```python
from build123d import *

# Parameters (mm, degrees)
SKETCH_3_R               = 3
EXTRUDE_6_DEPTH          = 0.001
EXTRUDE_6_2_DEPTH        = 0.001
EXTRUDE_6_3_DEPTH        = 0.001
EXTRUDE_6_4_DEPTH        = 0.001
CUT_EXTRUDE_2_DEPTH      = 67.213034483
CUT_EXTRUDE_2_DEPTH_BACK = 67.213034483
SKETCH_11_R              = 2.25
EXTRUDE_7_DEPTH          = 2
EXTRUDE_7_DEPTH_BACK     = 0.801922547
SKETCH_14_R              = 10
CUT_EXTRUDE_3_DEPTH      = 3
SKETCH_12_4_R            = 10
EXTRUDE_10_DEPTH         = 44
SKETCH_20_W              = 40.801922547
SKETCH_20_H              = 50
CUT_EXTRUDE_6_DEPTH      = 60
SKETCH_21_W              = 44.801922547
SKETCH_21_H              = 50
EXTRUDE_11_DEPTH         = 2
SKETCH_23_W              = 4
SKETCH_23_H              = 35
EXTRUDE_12_DEPTH         = 35
CUT_EXTRUDE_7_DEPTH      = 75.778269065
SKETCH_25_R              = 0.75
CUT_EXTRUDE_8_DEPTH      = 84.687483396
FILLET_2_R               = 5
FILLET_3_R               = 5
FILLET_5_R               = 3
FILLET_6_R               = 3
FILLET_7_R               = 3
FILLET_8_R               = 3
SKETCH_26_R              = 2.75
CUT_EXTRUDE_9_DEPTH      = 100
SKETCH_27_R              = 10
SKETCH_27_R_2            = 7.5
EXTRUDE_13_DEPTH         = 5
SKETCH_28_R              = 10
SKETCH_28_R_2            = 7.5
EXTRUDE_14_DEPTH         = 5
CUT_EXTRUDE_10_DEPTH     = 86.331157337
CUT_EXTRUDE_11_DEPTH     = 86.331157337
CUT_EXTRUDE_12_DEPTH     = 86.331157337
EXTRUDE_15_DEPTH         = 50


with BuildPart() as part:
    # Sketch 3 → Extrude 6 (new body)
    with BuildSketch(Plane.XY):
        with Locations((60.266478541, 16.532501821)):
            Circle(SKETCH_3_R)
    extrude(amount=EXTRUDE_6_DEPTH)


with BuildPart() as body_2:
    # Sketch 3 → Extrude 6 2 (new body)
    with BuildSketch(Plane.XY):
        with Locations((60.266478541, 6.532501821)):
            Circle(SKETCH_3_R)
    extrude(amount=EXTRUDE_6_2_DEPTH)


with BuildPart() as body_3:
    # Sketch 3 → Extrude 6 3 (new body)
    with BuildSketch(Plane.XY):
        with Locations((10.766478541, 6.532501821)):
            Circle(SKETCH_3_R)
    extrude(amount=EXTRUDE_6_3_DEPTH)


with BuildPart() as body_4:
    # Sketch 3 → Extrude 6 4 (new body)
    with BuildSketch(Plane.XY):
        with Locations((10.766478541, 16.532501821)):
            Circle(SKETCH_3_R)
    extrude(amount=EXTRUDE_6_4_DEPTH)


with BuildPart() as cut_extrude_2_tool:
    # Sketch 11 → Cut-Extrude 2 (new, two sides: drawn at the far end of the back side and taken through both)
    with BuildSketch(Plane.XY.offset(0.001).offset(-CUT_EXTRUDE_2_DEPTH_BACK)):
        with Locations((10.766478541, 16.532501821)):
            Circle(SKETCH_11_R)
        with Locations((10.766478541, 6.532501821)):
            Circle(SKETCH_11_R)
        with Locations((60.266478541, 16.532501821)):
            Circle(SKETCH_11_R)
        with Locations((60.266478541, 6.532501821)):
            Circle(SKETCH_11_R)
    extrude(amount=CUT_EXTRUDE_2_DEPTH + CUT_EXTRUDE_2_DEPTH_BACK)


with BuildPart() as part_1:
    add(part.part)

    # Cut-Extrude 2: cut by cut_extrude_2_tool
    add(cut_extrude_2_tool.part, mode=Mode.SUBTRACT)



with BuildPart() as body_2_1:
    add(body_2.part)

    # Cut-Extrude 2: cut by cut_extrude_2_tool
    add(cut_extrude_2_tool.part, mode=Mode.SUBTRACT)


with BuildPart() as body_3_1:
    add(body_3.part)

    # Cut-Extrude 2: cut by cut_extrude_2_tool
    add(cut_extrude_2_tool.part, mode=Mode.SUBTRACT)


with BuildPart() as body_4_1:
    add(body_4.part)

    # Cut-Extrude 2: cut by cut_extrude_2_tool
    add(cut_extrude_2_tool.part, mode=Mode.SUBTRACT)


with BuildPart() as body_5:
    # Sketch 12 → Extrude 7 (new, two sides: drawn at the far end of the back side and taken through both)
    with BuildSketch(Plane.XY.offset(0.001).offset(-EXTRUDE_7_DEPTH_BACK)):
        Polygon((5.516478541, 26.532501821), (65.516478541, 26.532501821), (65.516478541, -23.467498179), (5.516478541, -23.467498179), (5.516478541, 1.532501821), align=None)
    extrude(amount=EXTRUDE_7_DEPTH + EXTRUDE_7_DEPTH_BACK)

    # Sketch 14 → Cut-Extrude 3 (cut)
    with BuildSketch(Plane(origin=(0, 0, -0.800922547), x_dir=(-1, 0, 0), z_dir=(0, 0, -1))):
        with Locations((-45.516478541, 11.532501821)):
            Circle(SKETCH_14_R)
    extrude(amount=-CUT_EXTRUDE_3_DEPTH, mode=Mode.SUBTRACT)


with BuildPart() as part_2:
    add(part_1.part)

    add(body_2_1.part)  # Extrude 10 merges body 2

    add(body_3_1.part)  # Extrude 10 merges body 3

    add(body_4_1.part)  # Extrude 10 merges body 4

    add(body_5.part)  # Extrude 10 merges body 5
    # Sketch 12_4 → Extrude 10 (add)
    with BuildSketch(Plane.XY.offset(0.001)):
        Polygon((5.516478541, 26.532501821), (65.516478541, 26.532501821), (65.516478541, -23.467498179), (5.516478541, -23.467498179), (5.516478541, 1.532501821), align=None)
        with Locations(Location((45.516478541, 11.532501821, 0), (0, 0, 180))):
            Circle(SKETCH_12_4_R, mode=Mode.SUBTRACT)
    extrude(amount=EXTRUDE_10_DEPTH)

    # Sketch 20 → Cut-Extrude 6 (cut)
    with BuildSketch(Plane(origin=(65.516478541, 0, 0), x_dir=(0, 0, -1), z_dir=(1, 0, 0))):
        with Locations((-21.600038727, 1.532501821)):
            Rectangle(SKETCH_20_W, SKETCH_20_H)
    extrude(amount=-CUT_EXTRUDE_6_DEPTH, mode=Mode.SUBTRACT)


with BuildPart() as cut_extrude_6_piece_1:
    # of the separate pieces the step leaves, piece 1, a body of its own (cut_extrude_6_pieces)
    add(part_2.part.solids().sort_by_distance((5.516478541, 26.532501821, 42.001))[0])



with BuildPart() as cut_extrude_6_piece_2:
    # of the separate pieces the step leaves, piece 2, a body of its own (cut_extrude_6_pieces)
    add(part_2.part.solids().sort_by_distance((5.516478541, 26.532501821, -0.800922547))[0])


with BuildPart() as cut_extrude_6_piece_1_1:
    add(cut_extrude_6_piece_1.part)

    add(cut_extrude_6_piece_2.part)  # Extrude 11 merges Cut-Extrude 6 piece 2
    # Sketch 21 → Extrude 11 (add)
    with BuildSketch(Plane.ZY.offset(-5.516478541)):
        with Locations((21.600038727, 1.532501821)):
            Rectangle(SKETCH_21_W, SKETCH_21_H)
    extrude(amount=EXTRUDE_11_DEPTH)

    # Sketch 23 → Extrude 12 (add)
    with BuildSketch(Plane.ZY.offset(-3.516478541)):
        with Locations((21.600038726, 1.532501821)):
            Rectangle(SKETCH_23_W, SKETCH_23_H)
    extrude(amount=EXTRUDE_12_DEPTH)

    # Sketch 24 → Cut-Extrude 7 (cut, through all)
    with BuildSketch(Plane.XY.offset(23.600038726)):
        Polygon((-13.983521459, 12.492501821), (-24.943676567, 1.532346713), (-13.983521459, -9.427808395), (-3.023366351, 1.532346713), align=None)
    extrude(amount=-CUT_EXTRUDE_7_DEPTH, mode=Mode.SUBTRACT)

    # Sketch 25 → Cut-Extrude 8 (cut, through all)
    with BuildSketch(Plane(origin=(0, 0, -0.800922547), x_dir=(-1, 0, 0), z_dir=(0, 0, -1))):
        with Locations((-33.016478541, 19.032501821)):
            Circle(SKETCH_25_R)
        with Locations((-33.016478541, 4.032501821)):
            Circle(SKETCH_25_R)
        with Locations((-18.016478541, 19.032501821)):
            Circle(SKETCH_25_R)
        with Locations((-18.016478541, 3.622989742)):
            Circle(SKETCH_25_R)
        with Locations((-25.516478541, 19.032501821)):
            Circle(SKETCH_25_R)
        with Locations((-25.516478541, 3.827745781)):
            Circle(SKETCH_25_R)
        with Locations((-18.016478541, 11.327745781)):
            Circle(SKETCH_25_R)
    extrude(amount=-CUT_EXTRUDE_8_DEPTH, mode=Mode.SUBTRACT)

    # Fillet 2
    fillet_2_edges = [cut_extrude_6_piece_1_1.edges().sort_by_distance(p)[0] for p in [
        (65.516478541, 26.532501821, 0.199077453),
    ]]
    fillet(fillet_2_edges, radius=FILLET_2_R)

    # Fillet 3
    fillet_3_edges = [cut_extrude_6_piece_1_1.edges().sort_by_distance(p)[0] for p in [
        (65.516478541, 26.532501821, 43.001),
    ]]
    fillet(fillet_3_edges, radius=FILLET_3_R)

    # Fillet 5
    fillet_5_edges = [cut_extrude_6_piece_1_1.edges().sort_by_distance(p)[0] for p in [
        (3.516478541, 1.532501821, 44.001),
    ]]
    fillet(fillet_5_edges, radius=FILLET_5_R)

    # Fillet 6
    fillet_6_edges = [cut_extrude_6_piece_1_1.edges().sort_by_distance(p)[0] for p in [
        (3.516478541, 1.532501821, -0.800922547),
    ]]
    fillet(fillet_6_edges, radius=FILLET_6_R)

    # Fillet 7
    fillet_7_edges = [cut_extrude_6_piece_1_1.edges().sort_by_distance(p)[0] for p in [
        (-31.483521459, -15.967498179, 21.600038726),
    ]]
    fillet(fillet_7_edges, radius=FILLET_7_R)

    # Fillet 8
    fillet_8_edges = [cut_extrude_6_piece_1_1.edges().sort_by_distance(p)[0] for p in [
        (-31.483521459, 19.032501821, 21.600038726),
    ]]
    fillet(fillet_8_edges, radius=FILLET_8_R)

    # Sketch 26 → Cut-Extrude 9 (cut)
    with BuildSketch(Plane(origin=(0, 0, -0.800922547), x_dir=(-1, 0, 0), z_dir=(0, 0, -1))):
        with Locations((-24.586117818, -9.397858902)):
            Circle(SKETCH_26_R)
    extrude(amount=-CUT_EXTRUDE_9_DEPTH, mode=Mode.SUBTRACT)

    # Sketch 27 → Extrude 13 (add)
    with BuildSketch(Plane.XY.offset(1.199077453)):
        with Locations((24.586117818, -9.397858902)):
            Circle(SKETCH_27_R)
        with Locations((24.586117818, -9.397858902)):
            Circle(SKETCH_27_R_2, mode=Mode.SUBTRACT)
    extrude(amount=-EXTRUDE_13_DEPTH)

    # Sketch 28 → Extrude 14 (add)
    with BuildSketch(Plane(origin=(0, 0, 42.001), x_dir=(-1, 0, 0), z_dir=(0, 0, -1))):
        with Locations(Location((-24.586117818, -9.397858902, 0), (0, 0, 180))):
            Circle(SKETCH_28_R)
        with Locations(Location((-24.586117818, -9.397858902, 0), (0, 0, 180))):
            Circle(SKETCH_28_R_2, mode=Mode.SUBTRACT)
    extrude(amount=-EXTRUDE_14_DEPTH)

    # Sketch 29 → Cut-Extrude 10 (cut, through all)
    with BuildSketch(Plane(origin=(0, 0, -0.800922547), x_dir=(-1, 0, 0), z_dir=(0, 0, -1))):
        Polygon((-65.516478541, 4.105503733), (-36.016478541, -23.467498179), (-65.516478541, -23.467498179), align=None)
    extrude(amount=-CUT_EXTRUDE_10_DEPTH, mode=Mode.SUBTRACT)

    # Sketch 31 → Cut-Extrude 11 (cut, through all)
    with BuildSketch(Plane(origin=(0, 0, -0.800922547), x_dir=(-1, 0, 0), z_dir=(0, 0, -1))):
        with BuildLine():
            Line((-36.016478541, -23.467498179), (-38.899128386, -20.773148698))
            ThreePointArc((-38.899128386, -20.773148698), (-35.741085253, -22.769554543), (-32.070697344, -23.467498179))
            Line((-32.070697344, -23.467498179), (-36.016478541, -23.467498179))
        make_face()
    extrude(amount=-CUT_EXTRUDE_11_DEPTH, mode=Mode.SUBTRACT)

    # Sketch 32 → Cut-Extrude 12 (cut, through all)
    with BuildSketch(Plane(origin=(0, 0, -0.800922547), x_dir=(-1, 0, 0), z_dir=(0, 0, -1))):
        with BuildLine():
            Line((-65.516478541, 8.446758423), (-65.516478541, 4.105503733))
            Line((-65.516478541, 4.105503733), (-62.344909583, 1.141107904))
            ThreePointArc((-62.344909583, 1.141107904), (-64.689381855, 4.46456747), (-65.516478541, 8.446758423))
        make_face()
    extrude(amount=-CUT_EXTRUDE_12_DEPTH, mode=Mode.SUBTRACT)

    # Sketch 35 → Extrude 15 (add)
    with BuildSketch(Plane.XZ.offset(23.467498179)):
        Polygon((5.516478541, 42.001), (10.516478541, 42.001), (5.516478541, 37.001), align=None)
        Polygon((5.516478541, 1.199077453), (5.516478541, 6.199077453), (10.516478541, 1.199077453), align=None)
    extrude(amount=-EXTRUDE_15_DEPTH)


solid = cut_extrude_6_piece_1_1.part
```
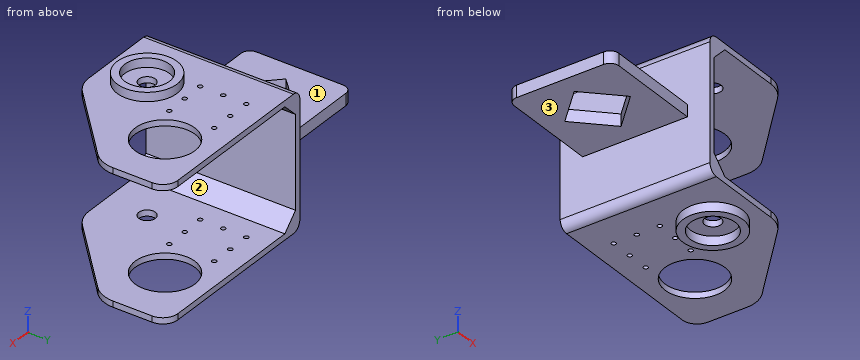
Here's how the part is built. I have some questions about the finished solid (model axes, mm). Face numbers are marked on the shaded views. Coordinates: 2 decimals unless noted, no trailing zeros. Order: outer loops, then holes, each group sorted by start corner. A loop starts at its lowest first (then second) coordinate and runs counter-clockwise, first axis right, second up. Notation, with made-up numbers: M -27.75,0.25 L 30.25,0.25 A12 ccw 30.25,22.25 Z; hole C -9.5,89 d10. An arc over 180 degrees is marked long. Answer as a JSON object with one key per item and string values. Group by question number.
(1) I need wall thicknesses on probe 1 along Z at (x, y) = (13.5, 15); probe 2 along X at (y, z) = (20, 36.5); probe 3 along Z at (x, y) = (-6.5, -4.5). Which ranges of each line are inside material? Lowest first, please.
(2) Suppose I cut it at B-B, the plane z = 22. Please give me the cut outline in (x, y).
(3) For pin 1 (10 mm diameter, centred on x = -11.5, y = 13.5, fed in from +Z); pin 2 (7 mm diameter, centred on x = 24.59, y = -9.4, fed in from -Z); pin 3 (1.4 mm diameter, centred on x = 18.02, y = 11.33, fed in from -Z); pin 4 (10 mm diameter, centred on x = -20.5, y = -7, fed in from -Z), each with a flat end and sliding along its axis, tell me the tip position at first contact or that it passes through.
(4) Suppose I cut it at C-C, the plane x = 41. Please give me the cut outline in (y, z), then the cut area to 3 significant figures.
(5) Suppose I cut it at D-D, the plane y = -10.5. State how many separate pieces and enclosed holes the cut face has, then the cut area to 3 significant figures.
(6) Suppose I cut it at A-A, the plane x = -8. Please give me the cut outline in (y, z), then the cut area to 3 significant figures.
(7) If we mould it in two halves opening along Z, with no side actions, what happens to the marked faces 1, 2 and 3? For each: released by +Z, released by -Z, zero draft, split by the parting line, or undercut.
Values found:
{
 "1": {"probe 1": "z = -0.8 to 1.2, 42 to 44", "probe 2": "x = 3.52 to 5.52", "probe 3": "z = 19.6 to 23.6"},
 "2": {"outline": "M -31.48,-12.97 A3 ccw -28.48,-15.97 L 3.52,-15.97 L 3.52,-23.47 L 5.52,-23.47 L 5.52,26.53 L 3.52,26.53 L 3.52,19.03 L -28.48,19.03 A3 ccw -31.48,16.03 Z; hole M -24.94,1.53 L -13.98,-9.43 L -3.02,1.53 L -13.98,12.49 Z"},
 "3": {"pin 1": "stops at z = 23.6", "pin 2": "stops at z = -0.8", "pin 3": "passes through", "pin 4": "stops at z = 19.6"},
 "4": {"outline": "M -18.81,-0.8 L 2.61,-0.8 L 2.61,1.2 L -18.81,1.2 Z; M -18.81,42 L 2.61,42 L 2.61,44 L -18.81,44 Z; M 20.45,-0.8 L 26.53,-0.8 L 26.53,1.2 L 20.45,1.2 Z; M 20.45,42 L 26.53,42 L 26.53,44 L 20.45,44 Z", "area": "110 mm^2"},
 "5": {"separate pieces": "3", "enclosed holes": "0", "area": "438 mm^2"},
 "6": {"outline": "M -15.97,19.6 L -3.44,19.6 L -3.44,23.6 L -15.97,23.6 Z; M 6.51,19.6 L 19.03,19.6 L 19.03,23.6 L 6.51,23.6 Z", "area": "100 mm^2"},
 "7": {"face 1": "released by +Z", "face 2": "undercut", "face 3": "released by -Z"}
}
